Check sheet for the modelled part. Datum: model origin and axes. Units: mm. Round coordinates to 2 decimals unless told otherwise and drop trailing zeros. Order: outer loops, then holes, each group sorted by start corner. A loop starts at its lowest first (then second) coordinate and runs counter-clockwise, first axis right, second up.
(1) Depth check by flat-ended pin: pin 1 (1.5 mm diameter, centred on y = 1, z = -1.5, fed in from +X); pin 2 (2 mm diameter, centred on x = 1, z = 121.5, fed in from +Y); pin 3 (5 mm diameter, centred on y = -4, z = 98.5, fed in from -X). Enter the tip coordinate at first touch or a pass-through.
(2) Sectioned sample at B-B, the plane y = 0. Enter the section's corners in (x, z), and give its area (3 significant figures).
(3) Sectioned sample at C-C, the plane z = 55.5. Enter the section's corners in (x, y), and give its area (3 significant figures).
(4) Sectioned sample at A-A, the plane x = 0.25. Enter the section's corners in (y, z).
(5) Thickness scan on probe 1 along Z at (x, y) = (0.75, -4); probe 2 along Y at (x, z) = (-2.75, 53); probe 3 along X at (y, z) = (0, 35.5). Record the ranges inside material, lowest first.
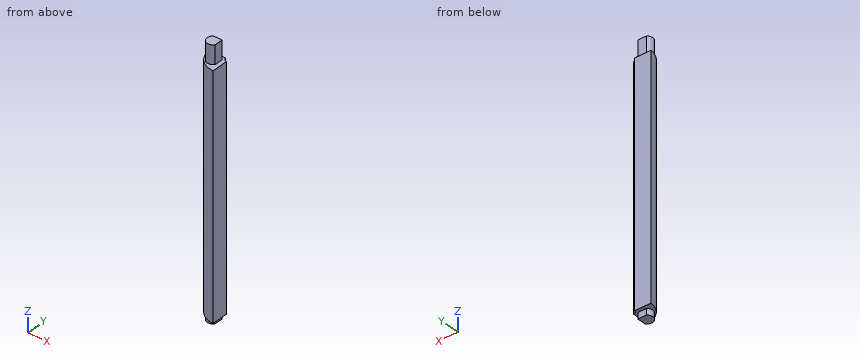
```python
from build123d import *

# Parameters (mm, degrees)
BOSS_EXTRUDE1_DEPTH      = 115
BOSS_EXTRUDE2_DEPTH      = 9
BOSS_EXTRUDE2_DEPTH_BACK = 118


with BuildPart() as part:
    # Sketch1 → Boss-Extrude1 (new body)
    with BuildSketch(Plane.XY):
        with BuildLine():
            Line((4.673790886, -4.96994292), (4.494306077, 3.000557085))
            ThreePointArc((4.494306077, 3.000557085), (3.322885957, 3.518832419), (2.673764356, 4.623131094))
            Line((2.673764356, 4.623131094), (-5.326209114, 4.643733806))
            ThreePointArc((-5.326209114, 4.643733806), (-2.250970398, -2.165211908), (4.673790886, -4.96994292))
        make_face()
    extrude(amount=BOSS_EXTRUDE1_DEPTH)

    # Sketch2 → Boss-Extrude2 (add, two sides: drawn at the far end of the back side and taken through both)
    with BuildSketch(Plane.XY.offset(115).offset(-BOSS_EXTRUDE2_DEPTH_BACK)):
        with BuildLine():
            Line((-1.673644669, 2.929860911), (2.526355331, 2.929860911))
            Line((2.526355331, 2.929860911), (2.526355331, -1.270139089))
            ThreePointArc((2.526355331, -1.270139089), (-2.001840649, -1.598335069), (-1.673644669, 2.929860911))
        make_face()
    extrude(amount=BOSS_EXTRUDE2_DEPTH + BOSS_EXTRUDE2_DEPTH_BACK)


solid = part.part
```
Derived:
1. pin 1: stops at x = 2.53
1. pin 2: stops at y = 2.93
1. pin 3: stops at x = -2.88
2. outline: (-3.96, 0) - (-2.83, 0) - (-2.83, -3) - (2.53, -3) - (2.53, 0) - (4.56, 0) - (4.56, 115) - (2.53, 115) - (2.53, 124) - (-2.83, 124) - (-2.83, 115) - (-3.96, 115) - close
2. area: 1,040 mm2
3. outline: (-5.33, 4.64) arc R10.05 ccw to (4.67, -4.97) - (4.49, 3) arc R2.09 cw to (2.67, 4.62) - close
3. area: 71.3 mm2
4. outline: (-3.92, 0) - (-2.47, 0) - (-2.47, -3) - (2.93, -3) - (2.93, 0) - (4.63, 0) - (4.63, 115) - (2.93, 115) - (2.93, 124) - (-2.47, 124) - (-2.47, 115) - (-3.92, 115) - close
5. probe 1: z = 0 to 115
5. probe 2: y = -1.65 to 4.64
5. probe 3: x = -3.96 to 4.56
